The listing builds one solid part. Answer for the finished solid, in the listing's coordinates (mm). Coordinates: 2 decimals unless noted, no trailing zeros. Write each loop counter-clockwise with the first axis right and the second up, starting at its lowest first coordinate (ties: lowest second). Pieces come first, ordered by that corner, then holes.
(1) The part is cut by section A-A on z = 4.25. Determine the outline of the cut face in (x, y), plus the area to 3 significant figures.
(2) The part is cut by section B-B on y = -5. Determine the outline of the cut face in (x, z), plus the area to 3 significant figures.
(3) Given P1, Ø4, axis at x = 3.5, z = -2, coming from the -Y side, flat-ended and moving along its own axis, determine where the tip first touches the part or whether it passes through.
(4) Straight lines are drawn through the part: line 1 (Z direction, x = -0.75, y = -0.25); line 2 (Y direction, x = 1.25, z = -1.25); line 3 (X direction, y = -2.75, z = 5). For each, find the intervals that lie inside material, in ascending order.
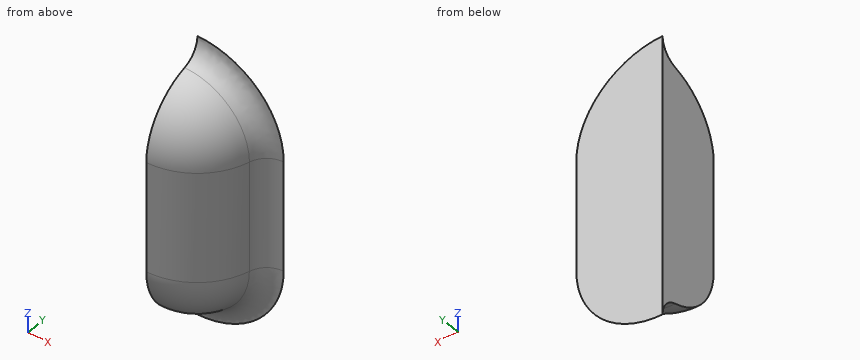
from build123d import *

# Parameters (mm, degrees)
SKETCH1_W           = 30
SKETCH1_H           = 3.464243611
BASE_EXTRUDE_DEPTH  = 25
BOSS_EXTRUDE1_DEPTH = 5
BOSS_REVOLVE2_ANGLE = 90
BOSS_REVOLVE3_ANGLE = 90
FILLET1_R           = 2
SKETCH8_W           = 50
SKETCH8_H           = 3.464243611
CUT_EXTRUDE4_DEPTH  = 40.509492685


with BuildPart() as part:
    # Sketch1 → Base-Extrude (new, symmetric)
    with BuildSketch(Plane.XY):
        with Locations((0, 1.732121806)):
            Rectangle(SKETCH1_W, SKETCH1_H)
    extrude(amount=BASE_EXTRUDE_DEPTH, both=True)

    # Louver Body → Boss-Extrude1 (add, symmetric)
    with BuildSketch(Plane.XY):
        with BuildLine():
            Line((-3, 0), (-3, -6))
            ThreePointArc((-3, -6), (1.242640687, -4.242640687), (3, 0))
            Line((3, 0), (-3, 0))
        make_face()
    extrude(amount=BOSS_EXTRUDE1_DEPTH, both=True)

    # Sketch12 → Boss-Revolve2 (revolve)
    with BuildSketch(Plane.XY.offset(5)):
        with BuildLine():
            Line((3, 0), (-3, 0))
            Line((-3, 0), (-3, -6))
            ThreePointArc((-3, -6), (1.242640687, -4.242640687), (3, 0))
        make_face()
    revolve(axis=Axis((-3, 0, 5), (0, -1, 0)), revolution_arc=BOSS_REVOLVE2_ANGLE)

    # Sketch13 → Boss-Revolve3 (revolve)
    with BuildSketch(Plane(origin=(0, 0, -5), x_dir=(-1, 0, 0), z_dir=(0, 0, -1))):
        with BuildLine():
            Line((3, 0), (-3, 0))
            ThreePointArc((-3, 0), (-1.242640687, -4.242640687), (3, -6))
            Line((3, -6), (3, 0))
        make_face()
    revolve(axis=Axis((-3, -6, -5), (0, 1, 0)), revolution_arc=BOSS_REVOLVE3_ANGLE)

    # Fillet1
    fillet1_edges = [part.edges().sort_by_distance(p)[0] for p in [
        (3, 0, 0),
        (1.242640687, 0, 9.242640687),
        (1.242640687, 0, -9.242640687),
    ]]
    fillet(fillet1_edges, radius=FILLET1_R)

    # Sketch8 → Cut-Extrude4 (cut, through all)
    with BuildSketch(Plane.ZY.offset(15)):
        with Locations((0, 1.732121806)):
            Rectangle(SKETCH8_W, SKETCH8_H)
    extrude(amount=-CUT_EXTRUDE4_DEPTH, mode=Mode.SUBTRACT)


solid = part.part
Model answer:
1. outline: (-3, -6) arc R6 ccw to (2.81, -1.5) arc R2 cw to (4.75, 0) - (-3, 0) - close
1. area: 28.8 mm2
2. outline: (-3, -8.32) arc R3.32 ccw to (0.32, -5) - (0.32, 5) arc R3.32 ccw to (-3, 8.32) - close
2. area: 50.4 mm2
3. P1: stops at y = -3.97
4. line 1: z = -11.39 to 11.39
4. line 2: y = -4.24 to 0
4. line 3: x = -3 to 2.33
